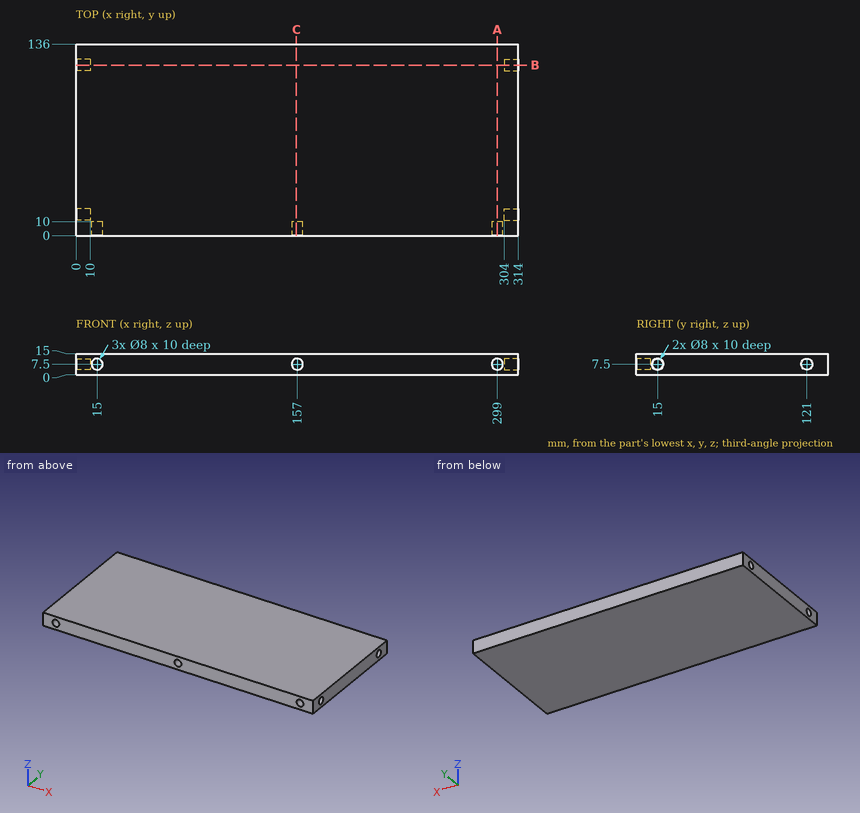
Study the drawing (mm; zero at the part's minimum x, y, z) and answer. Round coordinates to 2 decimals unless told otherwise and drop trailing zeros. Write each loop counter-clockwise with the first axis right and the second up, starting at its lowest first coordinate (ties: lowest second). Pieces come first, ordered by that corner, then holes. Notation, with made-up numbers: (1, -3) - (53, -3) arc R33 cw to (53, 28) - close; hole circle Ø6 at (46, 4). An arc over 180 degrees is marked (long way). Use a Markdown table: item, result. Add a question column.
1. The part is cut by section C-C (x = 156.5). Write down the section's boundary in (y, z), and give its area (3 significant figures).
2. The part is cut by section B-B (y = 121). Write down the section's boundary in (x, z), and give its area (3 significant figures).
3. The part is cut by section A-A (x = 299). Write down the section's boundary in (y, z).
4. Consider line 1 (Y direction, x = 7.5, z = 7.5); line 2 (Y direction, x = 15, z = 8). Determine where each line is inside the solid, lowest interval first.
5. Flat-ended cylindrical pins translate along their axes: P1, Ø2.5, axis at y = 122.5, z = 8.5, coming from the +X side; P2, Ø6.5, axis at x = 157, z = 7, coming from the -Y side; P3, Ø4, axis at y = 122.5, z = 7.5, coming from the -X side. Find the tip coordinate at first contact, or state that the pin passes through.
Reported:
| question | item | result |
|---|---|---|
| 1 | outline | (0, 0) - (136, 0) - (136, 15) - (0, 15) - (0, 11.47) - (10, 11.47) - (10, 3.53) - (0, 3.53) - close |
| 1 | area | 1,960 mm^2 |
| 2 | outline | (0, 0) - (314, 0) - (314, 3.5) - (304, 3.5) - (304, 11.5) - (314, 11.5) - (314, 15) - (0, 15) - (0, 11.5) - (10, 11.5) - (10, 3.5) - (0, 3.5) - close |
| 2 | area | 4,550 mm^2 |
| 3 | outline | (0, 0) - (136, 0) - (136, 15) - (0, 15) - (0, 11.5) - (10, 11.5) - (10, 3.5) - (0, 3.5) - close |
| 4 | line 1 | 0 to 11, 19 to 117, 125 to 136 |
| 4 | line 2 | 10 to 136 |
| 5 | P1 | x = 304 |
| 5 | P2 | y = 10 |
| 5 | P3 | x = 10 |
